```python
from build123d import *

# Parameters (mm, degrees)
CYLINDER007_R     = 2
CYLINDER007_DEPTH = 10
CYLINDER008_R     = 2
CYLINDER008_DEPTH = 10
CYLINDER009_R     = 2
CYLINDER009_DEPTH = 10
CYLINDER010_R     = 2
CYLINDER010_DEPTH = 10
CYLINDER006_R     = 2
CYLINDER006_DEPTH = 10
CYLINDER001_R     = 2
CYLINDER001_DEPTH = 10
CYLINDER005_R     = 2
CYLINDER005_DEPTH = 10
CYLINDER004_R     = 2
CYLINDER004_DEPTH = 10
CYLINDER003_R     = 2
CYLINDER003_DEPTH = 10
CYLINDER002_R     = 2
CYLINDER002_DEPTH = 10
CYLINDER_R        = 2
CYLINDER_DEPTH    = 10
PAD_DEPTH         = 3


with BuildPart() as cylinder007:
    # Cylinder007 → Cylinder007 (new body)
    with BuildSketch(Plane(origin=(117.5, 3.5, -3), x_dir=(1, 0, 0), z_dir=(0, 0, 1))):
        Circle(CYLINDER007_R)
    extrude(amount=CYLINDER007_DEPTH)


with BuildPart() as cylinder008:
    # Cylinder008 → Cylinder008 (new body)
    with BuildSketch(Plane(origin=(68.5, 3.5, -3), x_dir=(1, 0, 0), z_dir=(0, 0, 1))):
        Circle(CYLINDER008_R)
    extrude(amount=CYLINDER008_DEPTH)


with BuildPart() as cylinder009:
    # Cylinder009 → Cylinder009 (new body)
    with BuildSketch(Plane(origin=(17.5, 3.5, -3), x_dir=(1, 0, 0), z_dir=(0, 0, 1))):
        Circle(CYLINDER009_R)
    extrude(amount=CYLINDER009_DEPTH)


with BuildPart() as cylinder010:
    # Cylinder010 → Cylinder010 (new body)
    with BuildSketch(Plane(origin=(-31.5, 3.5, -3), x_dir=(1, 0, 0), z_dir=(0, 0, 1))):
        Circle(CYLINDER010_R)
    extrude(amount=CYLINDER010_DEPTH)


with BuildPart() as cylinder006:
    # Cylinder006 → Cylinder006 (new body)
    with BuildSketch(Plane(origin=(166.5, 3.5, -3), x_dir=(1, 0, 0), z_dir=(0, 0, 1))):
        Circle(CYLINDER006_R)
    extrude(amount=CYLINDER006_DEPTH)


with BuildPart() as cylinder001:
    # Cylinder001 → Cylinder001 (new body)
    with BuildSketch(Plane(origin=(166.5, -19, -3), x_dir=(1, 0, 0), z_dir=(0, 0, 1))):
        Circle(CYLINDER001_R)
    extrude(amount=CYLINDER001_DEPTH)


with BuildPart() as cylinder005:
    # Cylinder005 → Cylinder005 (new body)
    with BuildSketch(Plane(origin=(198.5, -21, -3), x_dir=(1, 0, 0), z_dir=(0, 0, 1))):
        Circle(CYLINDER005_R)
    extrude(amount=CYLINDER005_DEPTH)


with BuildPart() as cylinder004:
    # Cylinder004 → Cylinder004 (new body)
    with BuildSketch(Plane(origin=(-31.5, -19, -3), x_dir=(1, 0, 0), z_dir=(0, 0, 1))):
        Circle(CYLINDER004_R)
    extrude(amount=CYLINDER004_DEPTH)


with BuildPart() as cylinder003:
    # Cylinder003 → Cylinder003 (new body)
    with BuildSketch(Plane(origin=(68.5, -19, -3), x_dir=(1, 0, 0), z_dir=(0, 0, 1))):
        Circle(CYLINDER003_R)
    extrude(amount=CYLINDER003_DEPTH)


with BuildPart() as cylinder002:
    # Cylinder002 → Cylinder002 (new body)
    with BuildSketch(Plane(origin=(117.5, -19, -3), x_dir=(1, 0, 0), z_dir=(0, 0, 1))):
        Circle(CYLINDER002_R)
    extrude(amount=CYLINDER002_DEPTH)


with BuildPart() as cylinder:
    # Cylinder → Cylinder (new body)
    with BuildSketch(Plane(origin=(17.5, -19, -3), x_dir=(1, 0, 0), z_dir=(0, 0, 1))):
        Circle(CYLINDER_R)
    extrude(amount=CYLINDER_DEPTH)


with BuildPart() as cut010:
    # Sketch → Pad (new body)
    with BuildSketch(Plane.XY):
        Polygon((-39.423556, 10.687065), (185.576444, 10.687065), (205.306578, -20.03617), (197.646134, -26.464046), (181.576444, -7.312935), (174.576444, -7.312935), (169.576444, -22.312935), (163.576444, -22.312935), (158.576444, -7.312935), (125.576444, -7.312935), (120.576444, -22.312935), (114.576444, -22.312935), (109.576444, -7.312935), (76.576444, -7.312935), (71.576444, -22.312935), (65.576444, -22.312935), (60.576444, -7.312935), (25.576444, -7.312935), (20.576444, -22.312935), (14.576444, -22.312935), (9.576444, -7.312935), (-23.423556, -7.312935), (-28.423556, -22.312935), (-34.423556, -22.312935), (-39.423556, -7.312935), align=None)
    extrude(amount=PAD_DEPTH)

    # Cut: cut Cylinder
    add(cylinder.part, mode=Mode.SUBTRACT)

    # Cut001: cut Cylinder002
    add(cylinder002.part, mode=Mode.SUBTRACT)

    # Cut002: cut Cylinder003
    add(cylinder003.part, mode=Mode.SUBTRACT)

    # Cut003: cut Cylinder004
    add(cylinder004.part, mode=Mode.SUBTRACT)

    # Cut004: cut Cylinder005
    add(cylinder005.part, mode=Mode.SUBTRACT)

    # Cut005: cut Cylinder001
    add(cylinder001.part, mode=Mode.SUBTRACT)

    # Cut006: cut Cylinder006
    add(cylinder006.part, mode=Mode.SUBTRACT)

    # Cut007: cut Cylinder010
    add(cylinder010.part, mode=Mode.SUBTRACT)

    # Cut008: cut Cylinder009
    add(cylinder009.part, mode=Mode.SUBTRACT)

    # Cut009: cut Cylinder008
    add(cylinder008.part, mode=Mode.SUBTRACT)

    # Cut010: cut Cylinder007
    add(cylinder007.part, mode=Mode.SUBTRACT)


solid = cut010.part
```
Geometry check sheet. Reference: the model listing, model coordinates, mm. A direction names the side the tool comes from. Coordinates: 2 decimals unless noted, no trailing zeros. Loops run counter-clockwise (first coordinate to the right, second up) from the corner with the lowest first, then second, coordinate; pieces in that order, holes last. Notation, with made-up numbers: (9, 29.25) -> (59, 29.25) arc R28 cw to (59, 48.25) -> close; hole circle Ø10 at (-10, 47.5). An arc over 180 degrees is marked (long way). Put each result on its own line as item: value.
1) Release check for a two-part mould opening along Y. For faces 1 (the cylindrical face through (-29.592, 4.101, 1.479)), 2 (the flat face through (12.111, -14.918, 1.479)), 3 (the flat face through (195.303, -4.459, 1.479)), 4 (the cylindrical face through (-29.592, -18.399, 1.479)) record: released by +Y, released by -Y, zero draft, split by the parting line, or undercut.
Result set:
face 1: undercut
face 2: released by -Y
face 3: released by +Y
face 4: undercut
2) Cross-section at A-A on x = 68.5. Record the boundary of the cut face in (y, z), plus the area to 3 significant figures.
Result set:
outline: (-22.31, 0) -> (-21, 0) -> (-21, 3) -> (-22.31, 3) -> close; (-17, 0) -> (1.5, 0) -> (1.5, 3) -> (-17, 3) -> close; (5.5, 0) -> (10.69, 0) -> (10.69, 3) -> (5.5, 3) -> close
area: 75.0 mm^2
3) Tool access check on faces 5 (the cylindrical face through (164.502, 3.588, 1.479)), 6 (the flat face through (-25.89, -14.71, 1.48)). Record the directions out of +Z, -Z, +X, -X, +Y, -Y that give a thin tool (end or side, any length) a straight path to the whole face; none if there is none.
Result set:
face 5: +Z, -Z
face 6: +Z, -Z, -Y
4) Gauge pin test, flat ends, axial feed: pin 1 Ø0.9 at (x, z) = (-32.5, 2) entering from -Y; pin 2 Ø1.5 at (y, z) = (-5.5, 1) entering from +X; pin 3 Ø0.9 at (x, z) = (176.5, 1) entering from -Y. Record the tip position at first contact, or that the pin passes through.
Result set:
pin 1: stops at y = -22.31
pin 2: stops at x = 196.45
pin 3: stops at y = -7.31
5) Cross-section at D-D on y = -11. Record the boundary of the cut face in (x, z).
Result set:
outline: (-38.19, 0) -> (-24.65, 0) -> (-24.65, 3) -> (-38.19, 3) -> close; (10.81, 0) -> (24.35, 0) -> (24.35, 3) -> (10.81, 3) -> close; (61.81, 0) -> (75.35, 0) -> (75.35, 3) -> (61.81, 3) -> close; (110.81, 0) -> (124.35, 0) -> (124.35, 3) -> (110.81, 3) -> close; (159.81, 0) -> (173.35, 0) -> (173.35, 3) -> (159.81, 3) -> close; (184.67, 0) -> (199.5, 0) -> (199.5, 3) -> (184.67, 3) -> close
6) Thickness scan on line 1 (Y direction, x = 166.5, z = 0.75); line 2 (X direction, y = -11.5, z = 1.15); line 3 (X direction, y = -11, z = 0.25). Record the ranges inside material, lowest first.
Result set:
line 1: y = -22.31 to -21, -17 to 1.5, 5.5 to 10.69
line 2: x = -38.03 to -24.82, 10.97 to 24.18, 61.97 to 75.18, 110.97 to 124.18, 159.97 to 173.18, 185.09 to 199.82
line 3: x = -38.19 to -24.65, 10.81 to 24.35, 61.81 to 75.35, 110.81 to 124.35, 159.81 to 173.35, 184.67 to 199.5
7) Cross-section at B-B on y = 3.5. Record the boundary of the cut face in (x, z), plus the area to 3 significant figures.
Result set:
outline: (-39.42, 0) -> (-33.5, 0) -> (-33.5, 3) -> (-39.42, 3) -> close; (-29.5, 0) -> (15.5, 0) -> (15.5, 3) -> (-29.5, 3) -> close; (19.5, 0) -> (66.5, 0) -> (66.5, 3) -> (19.5, 3) -> close; (70.5, 0) -> (115.5, 0) -> (115.5, 3) -> (70.5, 3) -> close; (119.5, 0) -> (164.5, 0) -> (164.5, 3) -> (119.5, 3) -> close; (168.5, 0) -> (190.19, 0) -> (190.19, 3) -> (168.5, 3) -> close
area: 629 mm^2
8) Cross-section at C-C on z = 1.85. Count the separate pieces of the cut face and the enclosed holes in it, plus the area to 3 significant figures.
Result set:
separate pieces: 1
enclosed holes: 11
area: 5,060 mm^2
